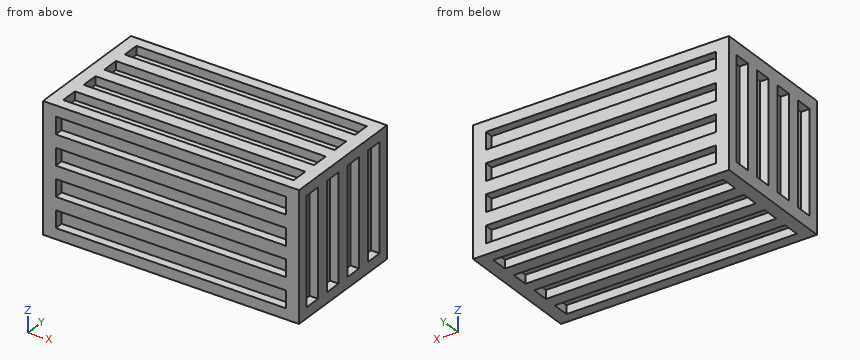
```python
from build123d import *

# Parameters (mm, degrees)
F0_W      = 60
F0_H      = 30
F1_DEPTH  = 30
F2_W      = 54
F2_H      = 4
F3_DEPTH  = 2
F4_W      = 54
F4_H      = 4
F5_DEPTH  = 2
F6_W      = 54
F6_H      = 4
F7_DEPTH  = 2
F8_W      = 54
F8_H      = 4
F9_DEPTH  = 2
F10_W     = 4
F10_H     = 24
F11_DEPTH = 2
F12_W     = 4
F12_H     = 25
F13_DEPTH = 2


with BuildPart() as f1:
    # F0 (on Front) → F1 (new body)
    with BuildSketch(Plane.XZ):
        Rectangle(F0_W, F0_H)
    extrude(amount=F1_DEPTH)

    # F2 (on face) → F3 (cut)
    with BuildSketch(Plane.XZ.offset(30)):
        with Locations((0, -10.5)):
            Rectangle(F2_W, F2_H)
        with Locations((0, -3.5)):
            Rectangle(F2_W, F2_H)
        with Locations((0, 3.5)):
            Rectangle(F2_W, F2_H)
        with Locations((0, 10.5)):
            Rectangle(F2_W, F2_H)
    extrude(amount=-F3_DEPTH, mode=Mode.SUBTRACT)

    # F4 (on face) → F5 (cut)
    with BuildSketch(Plane.XY.offset(15)):
        with Locations((0, -4.5)):
            Rectangle(F4_W, F4_H)
        with Locations((0, -11.5)):
            Rectangle(F4_W, F4_H)
        with Locations((0, -18.5)):
            Rectangle(F4_W, F4_H)
        with Locations((0, -25.5)):
            Rectangle(F4_W, F4_H)
    extrude(amount=-F5_DEPTH, mode=Mode.SUBTRACT)

    # F6 (on face) → F7 (cut)
    with BuildSketch(Plane(origin=(0, 0, 0), x_dir=(-1, 0, 0), z_dir=(0, 1, 0))):
        with Locations((0, 10.5)):
            Rectangle(F6_W, F6_H)
        with Locations((0, 3.5)):
            Rectangle(F6_W, F6_H)
        with Locations((0, -3.5)):
            Rectangle(F6_W, F6_H)
        with Locations((0, -10.5)):
            Rectangle(F6_W, F6_H)
    extrude(amount=-F7_DEPTH, mode=Mode.SUBTRACT)

    # F8 (on face) → F9 (cut)
    with BuildSketch(Plane(origin=(0, 0, -15), x_dir=(1, 0, 0), z_dir=(0, 0, -1))):
        with Locations((0, 25.5)):
            Rectangle(F8_W, F8_H)
        with Locations((0, 18.5)):
            Rectangle(F8_W, F8_H)
        with Locations((0, 11.5)):
            Rectangle(F8_W, F8_H)
        with Locations((0, 4.5)):
            Rectangle(F8_W, F8_H)
    extrude(amount=-F9_DEPTH, mode=Mode.SUBTRACT)

    # F10 (on face) → F11 (cut)
    with BuildSketch(Plane(origin=(-30, 0, 0), x_dir=(0, -1, 0), z_dir=(-1, 0, 0))):
        with Locations((4.5, 0)):
            Rectangle(F10_W, F10_H)
        with Locations((11.5, 0)):
            Rectangle(F10_W, F10_H)
        with Locations((18.5, 0)):
            Rectangle(F10_W, F10_H)
        with Locations((25.5, 0)):
            Rectangle(F10_W, F10_H)
    extrude(amount=-F11_DEPTH, mode=Mode.SUBTRACT)

    # F12 (on face) → F13 (cut)
    with BuildSketch(Plane.YZ.offset(30)):
        with Locations((-25.5, 0)):
            Rectangle(F12_W, F12_H)
        with Locations((-18.5, 0)):
            Rectangle(F12_W, F12_H)
        with Locations((-11.5, 0)):
            Rectangle(F12_W, F12_H)
        with Locations((-4.5, 0)):
            Rectangle(F12_W, F12_H)
    extrude(amount=-F13_DEPTH, mode=Mode.SUBTRACT)


solid = f1.part
```
Verification items for the finished model (mm, model axes). Coordinates: 2 decimals unless noted, no trailing zeros. Order: outer loops, then holes, each group sorted by start corner. A loop starts at its lowest first (then second) coordinate and runs counter-clockwise, first axis right, second up. Notation, with made-up numbers: (20, 16) -> (35, 16) arc R22 cw to (35, 33) -> close; hole circle Ø11 at (-34.75, 59.25). An arc over 180 degrees is marked (long way). Put each result on its own line as item: value. Start each with the question number.
1) Cross-section at A-A (y = -4.25). Enter the section's corners in (x, z), plus the area to 3 significant figures.
2) Go/stop test with flat-tipped pins: pin 1 (2 mm diameter, centred on x = -9, z = 14, fed in from +Y); pin 2 (1 mm diameter, centred on x = -14.5, y = -3.5, fed in from +Z); pin 3 (1.5 mm diameter, centred on x = 1, z = 10.5, fed in from +Y); pin 4 (1.2 mm diameter, centred on y = -24.5, z = -1, fed in from -X). Record where each tip stops, or that it passes through.
3) Material ranges on L1, parallel to Z at x = 23.5, y = -28.5; L2, parallel to Y at x = 13, z = -10; L3, parallel to Z at x = -12.5, y = -10.5, recorded low to high.
Geometry check:
1. outline: (-30, -15) -> (-27, -15) -> (-27, -13) -> (27, -13) -> (27, -15) -> (30, -15) -> (30, -12.5) -> (28, -12.5) -> (28, 12.5) -> (30, 12.5) -> (30, 15) -> (27, 15) -> (27, 13) -> (-27, 13) -> (-27, 15) -> (-30, 15) -> (-30, 12) -> (-28, 12) -> (-28, -12) -> (-30, -12) -> close
1. area: 1,490 mm^2
2. pin 1: stops at y = 0
2. pin 2: stops at z = 13
2. pin 3: stops at y = -2
2. pin 4: stops at x = -28
3. L1: z = -15 to -12.5, -8.5 to -5.5, -1.5 to 1.5, 5.5 to 8.5, 12.5 to 15
3. L2: y = -28 to -2
3. L3: z = -13 to 13
